Verification items for the finished model (mm, model axes). Face numbers are marked on the shaded views. A direction names the side the tool comes from. Give positions to 0.01 mm unless a question says otherwise; leave off trailing zeros. Order: outer loops, then holes, each group sorted by start corner. A loop starts at its lowest first (then second) coordinate and runs counter-clockwise, first axis right, second up. Notation, with made-up numbers: (49, -16.75) - (87, -16.75) arc R37 ccw to (87, 20.25) - close; hole circle Ø9 at (6, -15.75). An arc over 180 degrees is marked (long way). Answer as a JSON object with one key per item and string values.
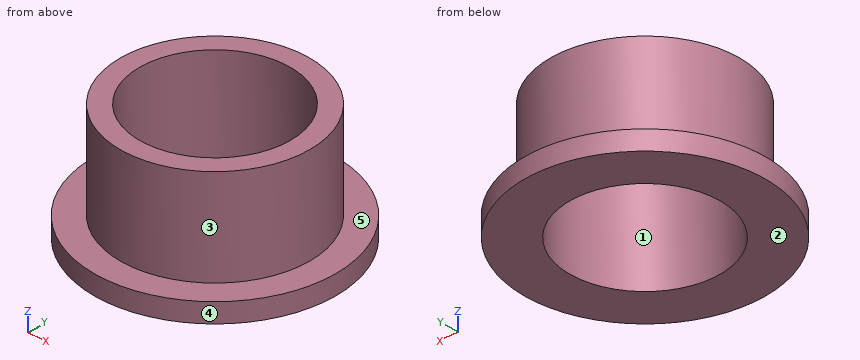
```python
from build123d import *

# Parameters (mm, degrees)
F0_R     = 24.887992
F1_DEPTH = 25.4
F2_R     = 31.71137
F3_DEPTH = 5.08
F4_R     = 19.832009
F5_DEPTH = 38.1


with BuildPart() as f1:
    # F0 (on Top) → F1 (new body)
    with BuildSketch(Plane.XY):
        Circle(F0_R)
    extrude(amount=F1_DEPTH)

    # F2 (on Top) → F3 (join)
    with BuildSketch(Plane.XY):
        Circle(F2_R)
    extrude(amount=-F3_DEPTH)

    # F4 (on face) → F5 (cut)
    with BuildSketch(Plane.XY.offset(25.4)):
        Circle(F4_R)
    extrude(amount=-F5_DEPTH, mode=Mode.SUBTRACT)


solid = f1.part
```
(1) Section check D-D (y = -22). Record the cut outline in (x, z), then the cut area to 3 significant figures.
Computed values:
{"outline": "(-22.84, -5.08) - (22.84, -5.08) - (22.84, 0) - (11.64, 0) - (11.64, 25.4) - (-11.64, 25.4) - (-11.64, 0) - (-22.84, 0) - close", "area": "823 mm²"}
(2) Release check for a two-part mould opening along Y. For the marked faces 1, 2 and 3 record: pulls with the +Y half, pulls with the -Y half, needs draft (parallel to the pull), parting line crosses it, or undercut.
Computed values:
{"face 1": "undercut", "face 2": "needs draft", "face 3": "parting line crosses it"}
(3) Material ranges on line 1 along Y through (x, z) = (0, 13); line 2 along Z through (x, y) = (-14, -24.5); line 3 along Y through (x, z) = (17.5, 0.5), recorded low to high. Write a range as [from, to].
Computed values:
{"line 1": "y = [-24.89, -19.83], [19.83, 24.89]", "line 2": "z = [-5.08, 0]", "line 3": "y = [-17.7, -9.33], [9.33, 17.7]"}
(4) Section check C-C (z = 13). Record the cut outline in (x, y).
Computed values:
{"outline": "circle Ø49.78 at (0, 0); hole circle Ø39.66 at (0, 0)"}
(5) Gauge pin test, flat ends, axial feed: pin 1 Ø10 at (x, z) = (3.5, 10.5) entering from +Y; pin 2 Ø3 at (x, z) = (16.5, 15.5) entering from -Y; pin 3 Ø10 at (x, z) = (7.5, 21.5) entering from +Y. Record the tip position at first contact, or that the pin passes through.
Computed values:
{"pin 1": "stops at y = 24.89", "pin 2": "stops at y = -19.86", "pin 3": "stops at y = 24.76"}
(6) Access from +Z, -Z, +X, -X, +Y, -Y to the whole of each face (thin tool, end or side, straight path). Record for the marked faces 4 and 5.
Computed values:
{"face 4": "+Z, -Z", "face 5": "+Z"}
(7) Section check A-A (x = 0). Record the cut outline in (y, z).
Computed values:
{"outline": "(-31.71, -5.08) - (-19.83, -5.08) - (-19.83, 25.4) - (-24.89, 25.4) - (-24.89, 0) - (-31.71, 0) - close; (19.83, -5.08) - (31.71, -5.08) - (31.71, 0) - (24.89, 0) - (24.89, 25.4) - (19.83, 25.4) - close"}
